The listing builds one solid part. Answer for the finished solid, in the listing's coordinates (mm). Face numbers are marked on the shaded views. Give positions to 0.01 mm unless a question says otherwise; leave off trailing zeros. Order: outer loops, then holes, each group sorted by start corner. A loop starts at its lowest first (then second) coordinate and runs counter-clockwise, first axis right, second up. Notation, with made-up numbers: (66.5, -4.75) -> (75.5, -4.75) arc R26 ccw to (75.5, 20.25) -> close; hole circle Ø2 at (-3.5, 61.25). An arc over 180 degrees is marked (long way). Answer as a JSON object with one key per item and string values. Group by question number.
```python
from build123d import *

# Parameters (mm, degrees)
BOSS_EXTRUDE2_DEPTH = 3.18


with BuildPart() as part:
    # Sketch3 → Boss-Extrude2 (new body)
    with BuildSketch(Plane.XY):
        with BuildLine():
            Line((154.566276863, 48.576), (126.154248002, 61.593943228))
            add(Edge.make_bspline(
                [(70.42492341, 64.420190492), (71.539940423, 64.519647115), (74.003845296, 64.716372581), (79.10872622, 65.136602193), (96.644785351, 66.182060474), (113.226942999, 66.103763633), (126.154248002, 61.593943228)],
                knots=[0.037653962, 0.037653962, 0.037653962, 0.037653962, 0.095230039, 0.164778525, 0.301013956, 1, 1, 1, 1], degree=3))
            add(Edge.make_bspline(
                [(69.748246193, 64.358453822), (69.973763165, 64.379520838), (70.199324622, 64.400067666), (70.42492341, 64.420190492)],
                knots=[0.026004729, 0.026004729, 0.026004729, 0.026004729, 0.037653962, 0.037653962, 0.037653962, 0.037653962], degree=3))
            add(Edge.make_bspline(
                [(58.782586434, 61.3879207), (59.955341201, 62.098447326), (61.681198084, 62.675723092), (64.027199959, 63.266819743), (66.422854867, 63.735360745), (68.36941666, 64.202932371), (69.748246193, 64.358453822)],
                knots=[0, 0, 0, 0, 0.338683805, 0.447560599, 0.600475936, 0.944024822, 0.944024822, 0.944024822, 0.944024822], degree=3))
            add(Edge.make_bspline(
                [(20.133826985, 48.853685786), (23.946969175, 49.456022002), (28.845183788, 49.969770281), (34.092791307, 50.505206975), (36.003857037, 50.880366768), (39.598247839, 51.906864384), (47.175860034, 55.732014815), (54.085013367, 59.506177314), (58.782586434, 61.3879207)],
                knots=[0, 0, 0, 0, 0.281454695, 0.359726601, 0.384533669, 0.423485214, 0.632085306, 1, 1, 1, 1], degree=3))
            add(Edge.make_bspline(
                [(9.07850141, 50.252079796), (14.251537818, 47.979183465), (20.133826985, 48.853685786)],
                knots=[0, 0, 0, 1, 1, 1], degree=2))
            Line((9.07850141, 50.252079796), (6.389579219, 49.571823086))
            Line((6.389579219, 49.571823086), (8.304869981, 45.881039625))
            Line((8.304869981, 45.881039625), (5.000125196, 34.613874444))
            Line((5.000125196, 34.613874444), (3.811505877, 34.339527184))
            Line((3.811505877, 34.339527184), (3.408141633, 30.275420379))
            Line((3.408141633, 30.275420379), (5.000125196, 23.378094633))
            Line((5.000125196, 23.378094633), (5.000125196, 19.880575438))
            Line((5.000125196, 19.880575438), (9.07850141, 15.370666667))
            Line((9.07850141, 15.370666667), (28.244198642, 10.740288968))
            Line((28.244198642, 10.740288968), (196.984326141, 11.285656733))
            Line((196.984326141, 11.285656733), (212.842666667, 13.119535563))
            Line((212.842666667, 13.119535563), (212.842666667, 14.278444622))
            Line((212.842666667, 14.278444622), (208.753166993, 15.166653328))
            Line((208.753166993, 15.166653328), (207.756612292, 16.09457661))
            Line((207.756612292, 16.09457661), (211.015778832, 22.30376088))
            add(Edge.make_bspline(
                [(213.311956775, 24.136094227), (213.208583455, 23.862222048), (212.957279088, 23.380062736), (212.30833351, 23.029337441), (211.606742708, 22.860432983), (211.183551066, 22.623391283), (211.015778832, 22.30376088)],
                knots=[0, 0, 0, 0, 0.295149858, 0.505508593, 0.707213933, 1, 1, 1, 1], degree=3))
            Line((213.311956775, 24.136094227), (213.311956775, 30.052431591))
            add(Edge.make_bspline(
                [(209.096417688, 31.906934109), (209.232301931, 31.198493688), (209.920582822, 30.680437528), (211.427560224, 29.98694305), (212.520853083, 30.088762434), (213.311956775, 30.052431591)],
                knots=[0, 0, 0, 0, 0.389815246, 0.499049524, 1, 1, 1, 1], degree=3))
            Line((209.096417688, 31.906934109), (209.096417688, 37.672126537))
            Line((209.096417688, 37.672126537), (210.346467514, 38.922176363))
            add(Edge.make_bspline(
                [(198.487796099, 43.845060743), (200.154143731, 43.736954664), (202.765045449, 43.082987453), (206.182994866, 42.256184747), (208.528724374, 40.831088376), (209.910383176, 39.742707025), (210.346467514, 38.922176363)],
                knots=[0, 0, 0, 0, 0.376788936, 0.61445489, 0.789914739, 1, 1, 1, 1], degree=3))
            Line((198.487796099, 43.845060743), (198.487796099, 46.439819769))
            add(Edge.make_bspline(
                [(197.590488958, 46.929659684), (197.958176787, 46.989526936), (198.336218206, 46.769514411), (198.487796099, 46.439819769)],
                knots=[0, 0, 0, 0, 1, 1, 1, 1], degree=3))
            Line((197.590488958, 46.929659684), (156.874666667, 48.576))
            Line((156.874666667, 48.576), (154.566276863, 48.576))
        make_face()
    extrude(amount=BOSS_EXTRUDE2_DEPTH)


solid = part.part
```
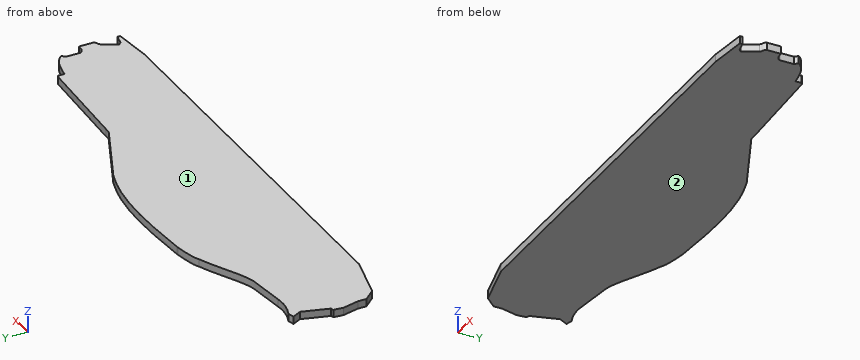
(1) For a pull along Z with two mould halves and no side action, classify the marked faces 1 and 2 as +Z half, -Z half, draft (parallel to the pull), parting line (faces both ways), or undercut.
(2) A cutting plane is placed at A-A (x = 162). Determine the outline of the cut face in (y, z).
(3) Find the intervals of material crossed by line 1 along Y through (x, z) = (150.5, 1.6); line 2 along X through (y, z) = (56.5, 1.75); line 3 along X through (y, z) = (20.5, 1.95), in increasing order. Write a range as [from, to].
(4) Flat-ended cylindrical pins translate along their axes: pin 1 Ø0.7 at (x, z) = (156, 1.5) entering from +Y; pin 2 Ø1.5 at (x, z) = (136, 1.5) entering from +Y; pin 3 Ø1.6 at (y, z) = (21, 2.5) entering from -X. Find the tip coordinate at first contact, or state that the pin passes through.
Check sheet entries:
{
 "1": {"face 1": "+Z half", "face 2": "-Z half"},
 "2": {"outline": "(11.17, 0) -> (48.37, 0) -> (48.37, 3.18) -> (11.17, 3.18) -> close"},
 "3": {"line 1": "y = [11.14, 50.44]", "line 2": "x = [48.51, 137.27]", "line 3": "x = [5, 210.07]"},
 "4": {"pin 1": "stops at y = 48.58", "pin 2": "stops at y = 57.43", "pin 3": "stops at x = 5"}
}
